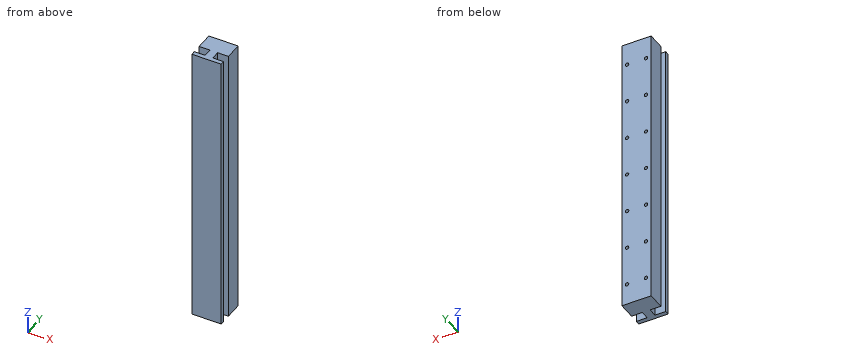
Autodesk Inventor part; units mm, degrees
ref_plane "YZ Plane" through (0, 0, 0) normal (1, 0, 0) x (0, 1, 0)
ref_plane "XZ Plane" through (0, 0, 0) normal (0, 1, 0) x (-1, 0, 0)
ref_plane "XY Plane" through (0, 0, 0) normal (0, 0, 1) x (1, 0, 0)
sketch "Эскиз1" plane through (0, 0, 0) normal (0, 0, 1) x (1, 0, 0)
  line L0 (0, 0) -> (68, 0)
  line L1 (68, 0) -> (68, -70)
  line L2 (68, -70) -> (0, -70)
  line L3 (0, -70) -> (0, 0)
  line L4 (0, 0) -> (0, -40)
  line L5 (0, -40) -> (25, -40)
  line L6 (25, -40) -> (25, -60)
  line L7 (25, -60) -> (0, -60)
  line L8 (34, 0) -> (34, -70)
  line L9 (68, -40) -> (43, -40)
  line L10 (43, -40) -> (43, -60)
  line L11 (43, -60) -> (68, -60)
  dimension "d0" = 68
  dimension "d1" = 70
  dimension "d2" = 40
  dimension "d3" = 25
  dimension "d4" = 20
extrude "Выдавливание1" add sketch "Эскиз1" along normal blind 660 contours L0 L8 L2 L3 L7 L6 L5 | L0 L1 L9 L10 L11 L2 L8
sketch "Эскиз2" plane through (0, 0, 0) normal (0, 1, 0) x (1, 0, 0)
  circle A0 centre (12, 10) radius 4
  line L0 (12, 10) -> (12, -50)
  point P0 (0, 0)
  dimension "d7" = 60
hole "Отверстие1" at (12, 0, 50) direction (0, -1, 0) diameter 6 depth 17 tip angle 118 counterbore diameter 8 counterbore depth 12
pattern_linear "Прямоуг.массив1" count 7 spacing 93 along (0, 0, 1) of "Отверстие1"
ref_plane "РабПлоскость1" through (34, -40, 0) normal (1, 0, 0) x (0, 0, -1)
mirror "Зеркальное отражение1" about plane through (34, -40, 0) normal (1, 0, 0) of "Отверстие1", "Прямоуг.массив1"
thread "Резьба1"
thread "Резьба2"
thread "Резьба3"
thread "Резьба4"
thread "Резьба5"
thread "Резьба6"
thread "Резьба7"
thread "Резьба8"
thread "Резьба9"
thread "Резьба10"
thread "Резьба11"
thread "Резьба12"
thread "Резьба13"
thread "Резьба14"
properties part number "Балка" material "Чугун, серый"
Geometry check sheet. Reference: the model listing, model coordinates, mm. Coordinates: 2 decimals unless noted, no trailing zeros. Order: outer loops, then holes, each group sorted by start corner. A loop starts at its lowest first (then second) coordinate and runs counter-clockwise, first axis right, second up. Notation, with made-up numbers: (14, 73.25) -> (21, 73.25) arc R15 ccw to (21, 79.25) -> close; hole circle Ø11 at (42, -4.5). An arc over 180 degrees is marked (long way). Use a Markdown table: item, result. Add a question column.
1. Cross-section at A-A (z = 546). Enter the section's corners in (x, y).
2. Go/stop test with flat-tipped pins: pin 1 Ø3.5 at (x, z) = (56, 422) entering from +Y; pin 2 Ø7 at (x, z) = (56, 236) entering from +Y; pin 3 Ø5.5 at (x, z) = (12, 143) entering from +Y. Record where each tip stops, or that it passes through.
3. Cross-section at B-B (y = -46). Enter the section's corners in (x, z), and give its area (3 significant figures).
4. Material ranges on L1, parallel to X at y = -9.25, z = 143; L2, parallel to X at y = -14.5, z = 329.5; L3, parallel to Y at x = 18.5, z = 621.5, recorded low to high.
Filled sheet:
| question | item | result |
|---|---|---|
| 1 | outline | (0, -70) -> (68, -70) -> (68, -60) -> (43, -60) -> (43, -40) -> (68, -40) -> (68, 0) -> (0, 0) -> (0, -40) -> (25, -40) -> (25, -60) -> (0, -60) -> close |
| 2 | pin 1 | y = -17.75 |
| 2 | pin 2 | y = -12 |
| 2 | pin 3 | y = -17.15 |
| 3 | outline | (25, 0) -> (43, 0) -> (43, 660) -> (25, 660) -> close |
| 3 | area | 11,900 mm2 |
| 4 | L1 | 0 to 8, 16 to 52, 60 to 68 |
| 4 | L2 | 0 to 9.04, 14.96 to 53.04, 58.96 to 68 |
| 4 | L3 | -70 to -60, -40 to 0 |
